from build123d import *

# Parameters (mm, degrees)
SKETCH_1_R          = 55
EXTRUDE_1_DEPTH     = 37.5
SKETCH_3_R          = 49.5
CUT_EXTRUDE_1_DEPTH = 32.5
SKETCH_5_W          = 43
SKETCH_5_H          = 12.242897151
CUT_EXTRUDE_2_DEPTH = 40
FILLET_4_R          = 2
FILLET_5_R          = 2
SKETCH_6_R          = 5
CUT_EXTRUDE_3_DEPTH = 12
EXTRUDE_START       = -5
EXTRUDE_3_DEPTH     = 5
FILLET_7_R          = 10
FILLET_8_R          = 5
SKETCH_10_R         = 3
CUT_EXTRUDE_5_DEPTH = 5
EXTRUDE_START_2     = 2.5
EXTRUDE_4_DEPTH     = 2.5
SKETCH_16_R         = 2
CUT_EXTRUDE_6_DEPTH = 10


with BuildPart() as part:
    # 草图1 → 凸台-拉伸1 (new body)
    with BuildSketch(Plane(origin=(0, 0, 0), x_dir=(1, 0, 0), z_dir=(0, 1, 0))):
        with Locations(Location((0, 0, 0), (0, 0, 270))):
            Circle(SKETCH_1_R)
    extrude(amount=EXTRUDE_1_DEPTH)

    # 草图3 → 切除-拉伸1 (cut)
    with BuildSketch(Plane(origin=(0, 37.5, 0), x_dir=(1, 0, 0), z_dir=(0, 1, 0))):
        with Locations(Location((0, 0, 0), (0, 0, 270))):
            Circle(SKETCH_3_R)
    extrude(amount=-CUT_EXTRUDE_1_DEPTH, mode=Mode.SUBTRACT)

    # 草图5 → 切除-拉伸2 (cut)
    with BuildSketch(Plane(origin=(0, 37.5, 0), x_dir=(1, 0, 0), z_dir=(0, 1, 0))):
        with Locations((0, 50.708442195)):
            Rectangle(SKETCH_5_W, SKETCH_5_H)
    extrude(amount=-CUT_EXTRUDE_2_DEPTH, mode=Mode.SUBTRACT)

    # 圆角4
    fillet_4_edges = [part.edges().sort_by_distance(p)[0] for p in [
        (-21.5, 18.75, -50.623611092),
    ]]
    fillet(fillet_4_edges, radius=FILLET_4_R)

    # 圆角5
    fillet_5_edges = [part.edges().sort_by_distance(p)[0] for p in [
        (21.5, 18.75, -50.623611092),
    ]]
    fillet(fillet_5_edges, radius=FILLET_5_R)

    # 草图6 → 切除-拉伸3 (cut)
    with BuildSketch(Plane(origin=(0, 5, 0), x_dir=(1, 0, 0), z_dir=(0, 1, 0))):
        with Locations(Location((0, 0, 0), (0, 0, 270))):
            Circle(SKETCH_6_R)
    extrude(amount=-CUT_EXTRUDE_3_DEPTH, mode=Mode.SUBTRACT)

    # 草图14 → 凸台-拉伸3 (add)
    with BuildSketch(Plane(origin=(0, 5, 0), x_dir=(1, 0, 0), z_dir=(0, 1, 0)).offset(EXTRUDE_START)):
        with BuildLine():
            Line((-49.898576095, 23.132922507), (-63.862525635, 37.044772973))
            Line((-63.862525635, 37.044772973), (-49.746845912, 51.213315099))
            Line((-49.746845912, 51.213315099), (-38.128637352, 39.638453724))
            ThreePointArc((-38.128637352, 39.638453724), (-44.78063998, 31.932652301), (-49.898576095, 23.132922507))
        make_face()
        with BuildLine():
            Line((49.811900188, -23.3189751), (64.421720913, -37.928795825))
            Line((64.421720913, -37.928795825), (50.279585289, -52.070931449))
            Line((50.279585289, -52.070931449), (37.984884655, -39.776230814))
            ThreePointArc((37.984884655, -39.776230814), (44.662950793, -32.097053236), (49.811900188, -23.3189751))
        make_face()
        with BuildLine():
            Line((-49.632393674, -23.698639164), (-63.862550335, -37.928795825))
            Line((-63.862550335, -37.928795825), (-49.720414711, -52.070931449))
            Line((-49.720414711, -52.070931449), (-37.697852746, -40.048369484))
            ThreePointArc((-37.697852746, -40.048369484), (-44.423770724, -32.427281642), (-49.632393674, -23.698639164))
        make_face()
        with BuildLine():
            Line((38.475737251, 39.301623923), (50.118901666, 51.212426922))
            Line((50.118901666, 51.212426922), (64.420808036, 37.231887798))
            Line((64.420808036, 37.231887798), (50.134465219, 22.6171483))
            ThreePointArc((50.134465219, 22.6171483), (45.083643676, 31.50341367), (38.475737251, 39.301623923))
        make_face()
    extrude(amount=EXTRUDE_3_DEPTH)

    # 圆角7
    fillet_7_edges = [part.edges().sort_by_distance(p)[0] for p in [
        (-38.128637352, 2.5, -39.638453724),
        (-49.898576095, 2.5, -23.132922507),
        (-49.632393674, 2.5, 23.698639164),
        (-37.697852746, 2.5, 40.048369484),
        (50.134465219, 2.5, -22.6171483),
        (38.475737251, 2.5, -39.301623923),
        (37.984884655, 2.5, 39.776230814),
        (49.811900188, 2.5, 23.3189751),
    ]]
    fillet(fillet_7_edges, radius=FILLET_7_R)

    # 圆角8
    fillet_8_edges = [part.edges().sort_by_distance(p)[0] for p in [
        (-63.862525635, 2.5, -37.044772973),
        (-49.746845912, 2.5, -51.213315099),
        (-49.720414711, 2.5, 52.070931449),
        (-63.862550335, 2.5, 37.928795825),
        (50.118901666, 2.5, -51.212426922),
        (64.420808036, 2.5, -37.231887798),
        (50.279585289, 2.5, 52.070931449),
        (64.421720913, 2.5, 37.928795825),
    ]]
    fillet(fillet_8_edges, radius=FILLET_8_R)

    # 草图10 → 切除-拉伸5 (cut)
    with BuildSketch(Plane(origin=(0, 5, 0), x_dir=(1, 0, 0), z_dir=(0, 1, 0))):
        with Locations(Location((-49.720414711, 37.071204175, 0), (0, 0, 270))):
            Circle(SKETCH_10_R)
        with Locations(Location((50.279585289, 37.071204175, 0), (0, 0, 270))):
            Circle(SKETCH_10_R)
        with Locations(Location((-49.720414711, -37.928795825, 0), (0, 0, 270))):
            Circle(SKETCH_10_R)
        with Locations(Location((50.279585289, -37.928795825, 0), (0, 0, 270))):
            Circle(SKETCH_10_R)
    extrude(amount=-CUT_EXTRUDE_5_DEPTH, mode=Mode.SUBTRACT)

    # 草图15 → 凸台-拉伸4 (add)
    with BuildSketch(Plane(origin=(0, 5, 0), x_dir=(1, 0, 0), z_dir=(0, 1, 0)).offset(EXTRUDE_START_2)):
        with BuildLine():
            Line((-21.5, 44.586993619), (-16.255768207, 44.586993619))
            ThreePointArc((-16.255768207, 44.586993619), (0, -47.457876059), (16.255768207, 44.586993619))
            Line((16.255768207, 44.586993619), (21.5, 44.586993619))
            ThreePointArc((21.5, 44.586993619), (0, -49.5), (-21.5, 44.586993619))
        make_face()
    extrude(amount=-EXTRUDE_4_DEPTH)

    # 草图16 → 切除-拉伸6 (cut)
    with BuildSketch(Plane(origin=(0, 0, 0), x_dir=(-1, 0, 0), z_dir=(0, -1, 0))):
        with Locations(Location((36, 0, 0), (0, 0, 90))):
            Circle(SKETCH_16_R)
        with Locations(Location((-36, 0, 0), (0, 0, 90))):
            Circle(SKETCH_16_R)
    extrude(amount=-CUT_EXTRUDE_6_DEPTH, mode=Mode.SUBTRACT)


solid = part.part
Read the model definition and answer for the solid it produces. Units are mm, in the model's axes. A direction names the side the tool comes from. Give positions to 0.01 mm unless a question says otherwise; leave off trailing zeros. Write each loop counter-clockwise with the first axis right and the second up, starting at its lowest first coordinate (ties: lowest second). Pieces come first, ordered by that corner, then holes. Notation, with made-up numbers: M -33.5,50.25 L -3.5,50.25 A16 cw -3.5,55.25 Z; hole C 42.5,86.25 d11. An arc over 180 degrees is marked long. One line per item, written item: value. Start each with the question number.
(1) Find the intervals of material crossed by line 1 (X direction, y = 1.8, z = 0); line 2 (Y direction, x = 12, z = -14); line 3 (X direction, y = 6.05, z = 0), in increasing order.
(2) Find section A-A (z = 0). Determine the outline of the cut face in (x, y), plus the area to 3 significant figures.
(3) Determine the mould class of faces 1 (the cylindrical face through (50.09, 2.54, -49.14)), 2 (the flat face through (-56.84, 2.46, 44.95)), 3 (the flat face through (57.22, 2.46, -44.27)) for opening direction X: pulls with the +X half, pulls with the -X half, needs draft (parallel to the pull), parting line crosses it, or undercut.
(4) Find section C-C (y = 17). Determine the outline of the cut face in (x, z).
(5) Find section B-B (x = 0). Determine the outline of the cut face in (y, z).
(6) Flat-ended cylindrical pins translate along their axes: pin 1 Ø4.5 at (x, z) = (36, 0) entering from +Y; pin 2 Ø0.9 at (y, z) = (23, -45.5) entering from +X; pin 3 Ø5 at (x, y) = (36.5, 8) entering from -Z; pin 4 Ø8 at (x, z) = (50.28, -37.07) entering from -Y. Find the tip coordinate at first contact, or state that the pin passes through.
(7) Find section D-D (x = 42). Determine the outline of the cut face in (y, z).
(8) A tool of negligible diameter and unlimited length cuts with its end or side. For faces 4 (the flat face through (47, 5, 37)), 5 (the cylindrical face through (34, 2, 0)), 6 (the flat face through (-52.3, 5, 39.9)), 7 (the cylindrical face through (-51.868, 2.535, -22.913)), 8 (the flat face through (-21.5, 19, -46)), from which of +Z, -Z, +X, -X, +Y, -Y can it reach the whole face along a straight path? Write none if from no direction.
Results below:
1. line 1: x = -55 to -38, -34 to -5, 5 to 34, 38 to 55
1. line 2: y = 0 to 5
1. line 3: x = -55 to -47.46, 47.46 to 55
2. outline: M -55,0 L -38,0 L -38,5 L -47.46,5 L -47.46,7.5 L -49.5,7.5 L -49.5,37.5 L -55,37.5 Z; M -34,0 L -5,0 L -5,5 L -34,5 Z; M 5,0 L 34,0 L 34,5 L 5,5 Z; M 38,0 L 55,0 L 55,37.5 L 49.5,37.5 L 49.5,7.5 L 47.46,7.5 L 47.46,5 L 38,5 Z
2. area: 828 mm^2
3. face 1: undercut
3. face 2: pulls with the -X half
3. face 3: pulls with the +X half
4. outline: M -24.39,-49.3 A2 ccw -21.5,-47.51 L -21.5,-44.59 A49.5 cw long 21.5,-44.59 L 21.5,-47.51 A2 ccw 24.39,-49.3 A55 ccw long Z
5. outline: M 0,-44.59 L 5,-44.59 L 5,-5 L 0,-5 Z; M 0,5 L 5,5 L 5,47.46 L 7.5,47.46 L 7.5,49.5 L 37.5,49.5 L 37.5,55 L 0,55 Z
6. pin 1: stops at y = 5
6. pin 2: stops at x = 31.55
6. pin 3: stops at z = -43.23
6. pin 4: stops at y = 0
7. outline: M 0,-43.83 L 5,-43.83 L 5,-35.51 L 37.5,-35.51 L 37.5,-26.2 L 7.5,-26.2 L 7.5,-22.1 L 5,-22.1 L 5,22.1 L 7.5,22.1 L 7.5,26.2 L 37.5,26.2 L 37.5,35.51 L 5,35.51 L 5,44.41 L 0,44.41 Z
8. face 4: +Z, +X, +Y
8. face 5: +Y, -Y
8. face 6: +Z, -X, +Y
8. face 7: -X, +Y, -Y
8. face 8: -Z, +Y, -Y
